```python
from build123d import *

# Parameters (mm, degrees)
F0_W           = 20
F0_H           = 20
F0_R           = 6
F0_R_2         = 5
F0_R_3         = 3.5
F1_DEPTH       = 5
F2_DEPTH       = 6
F3_DEPTH       = 1
F4_D           = 3.4
F4_START       = 1
F4_CSINK_D     = 6.72
F4_CSINK_ANGLE = 90
F6_ANGLE       = 180


# Not quite as in the source:
# - a fillet or chamfer that OpenCascade refuses, or shapes differently, is made with other operations: its cross-section is extruded or revolved along the edge and cut away or added


with BuildPart() as f1:
    # F0 (on Top) → F1 (new body)
    with BuildSketch(Plane.XY):
        Rectangle(F0_W, F0_H)
        Circle(F0_R, mode=Mode.SUBTRACT)
        Circle(F0_R)
        Circle(F0_R_2, mode=Mode.SUBTRACT)
        Circle(F0_R_2)
        Circle(F0_R_3, mode=Mode.SUBTRACT)
        Circle(F0_R_3)
    extrude(amount=-F1_DEPTH)

    # F0 (on Top) → F2 (join)
    with BuildSketch(Plane.XY):
        Circle(F0_R)
        Circle(F0_R_2, mode=Mode.SUBTRACT)
    extrude(amount=-F2_DEPTH)

    # F0 (on Top) → F3 (cut)
    with BuildSketch(Plane.XY):
        Circle(F0_R_3)
    extrude(amount=-F3_DEPTH, mode=Mode.SUBTRACT)

    # F4 (through all)
    # its depths count from where the whole tool has entered the part; down to there all is cleared
    with Locations(Plane.XY.offset(-F4_START)):
        with Locations((0, 0)):
            CounterSinkHole(F4_D / 2, F4_CSINK_D / 2, counter_sink_angle=F4_CSINK_ANGLE)

    # F5: fillet of radius 5 on 1 edges, made by hand

    # F5_s1 → F5_t2 (revolve)
    with BuildSketch(Plane.XZ):
        with BuildLine():
            ThreePointArc((9, -5), (7.4188611699, -5.2565835097), (6, -6))
            Line((6, -6), (5.94, -5.92))
            ThreePointArc((5.94, -5.92), (5.9, -5.5), (5.9, -5))
            Line((5.9, -5), (6, -4.9))
            Line((6, -4.9), (9, -4.9))
            Line((9, -4.9), (9, -5))
        make_face()
    revolve(axis=Axis((0, 0, -5), (0, 0, 1)))


with BuildPart() as f1_1:
    # F6: moved
    add(f1.part.rotate(Axis((0, 10, 0), (-1, 0, 0)), F6_ANGLE))


solid = f1_1.part
```
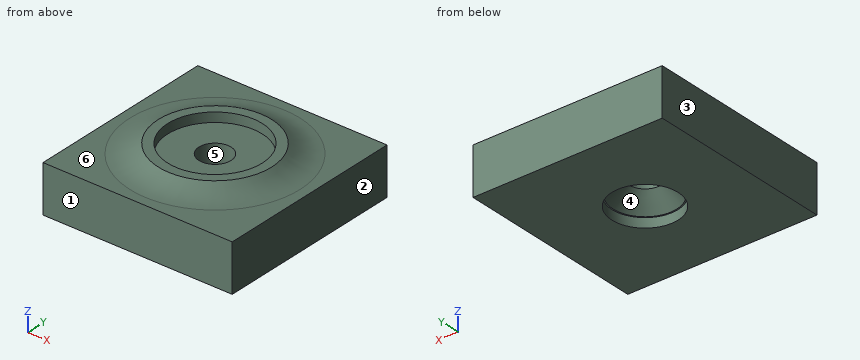
Model file for the job. Use its own axes, mm. Face numbers are marked on the shaded views. A direction names the side the tool comes from. Round coordinates to 2 decimals unless told otherwise and drop trailing zeros. Write each loop counter-clockwise with the first axis right and the second up, starting at its lowest first coordinate (ties: lowest second). Pieces come first, ordered by that corner, then holes. Notation, with made-up numbers: (15, 39.5) - (34, 39.5) arc R17 ccw to (34, 62.5) - close; hole circle Ø6 at (43, 29). An arc over 180 degrees is marked (long way). Use CSV: the item, a comma, the result in double quotes. Start each with the question number.
Item 1: Two-plate mould, pull along X, no slides. Class the marked faces 1, 2, 3 and 4: released by +X, released by -X, zero draft, split by the parting line, or undercut.
Item 2: Drill centre lines: L1, parallel to Y at x = 0, z = 0.4; L2, parallel to Y at x = 0, z = 4.55; L3, parallel to X at y = 20, z = 0.55. Where is each one in solid material? Low to high. Write a range as [from, to].
Item 3: Band-saw the part on C-C (x = 0). Write the cut outline in (y, z).
Item 4: Tool access for the marked faces 5 and 6: list every direction of +Z, -Z, +X, -X, +Y, -Y with a clear straight run to the whole face (end or side of a thin tool).
Item 5: Band-saw the part on A-A (y = 20). Write the cut outline in (x, z).
Item 6: Pin check, flat tip, straight feed: P1, Ø1, axis at x = -3.5, y = 20, coming from the +Z side. Stop position of the tip, or through.
Item 7: Band-saw the part on D-D (z = 2.25). Write the cut outline in (x, y).
Item 8: Band-saw the part on B-B (z = 3.5). Write the cut outline in (x, y), and give its area (3 significant figures).
Checked values:
1,face 1,"zero draft"
1,face 2,"released by +X"
1,face 3,"released by -X"
1,face 4,"undercut"
2,L1,"y = [10, 16.5], [23.5, 30]"
2,L2,"y = [10, 18.3], [21.7, 30]"
2,L3,"x = [-10, -3.5], [3.5, 10]"
3,outline,"(10, 0) - (16.5, 0) - (16.5, 1) - (16.64, 1) - (18.3, 2.66) - (18.3, 5) - (15, 5) - (15, 6) - (14, 6) arc R5 cw to (11, 5) - (10, 5) - close; (21.7, 2.66) - (23.36, 1) - (23.5, 1) - (23.5, 0) - (30, 0) - (30, 5) - (29, 5) arc R5 cw to (26, 6) - (25, 6) - (25, 5) - (21.7, 5) - close"
4,face 5,"+Z, -Z"
4,face 6,"+Z"
5,outline,"(-10, 0) - (-3.5, 0) - (-3.5, 1) - (-3.36, 1) - (-1.7, 2.66) - (-1.7, 5) - (-5, 5) - (-5, 6) - (-6, 6) arc R5 cw to (-9, 5) - (-10, 5) - close; (1.7, 2.66) - (3.36, 1) - (3.5, 1) - (3.5, 0) - (10, 0) - (10, 5) - (9, 5) arc R5 cw to (6, 6) - (5, 6) - (5, 5) - (1.7, 5) - close"
6,P1,"stops at z = 5"
7,outline,"(-10, 10) - (10, 10) - (10, 30) - (-10, 30) - close; hole circle Ø4.22 at (0, 20)"
8,outline,"(-10, 10) - (10, 10) - (10, 30) - (-10, 30) - close; hole circle Ø3.4 at (0, 20)"
8,area,"391 mm²"
